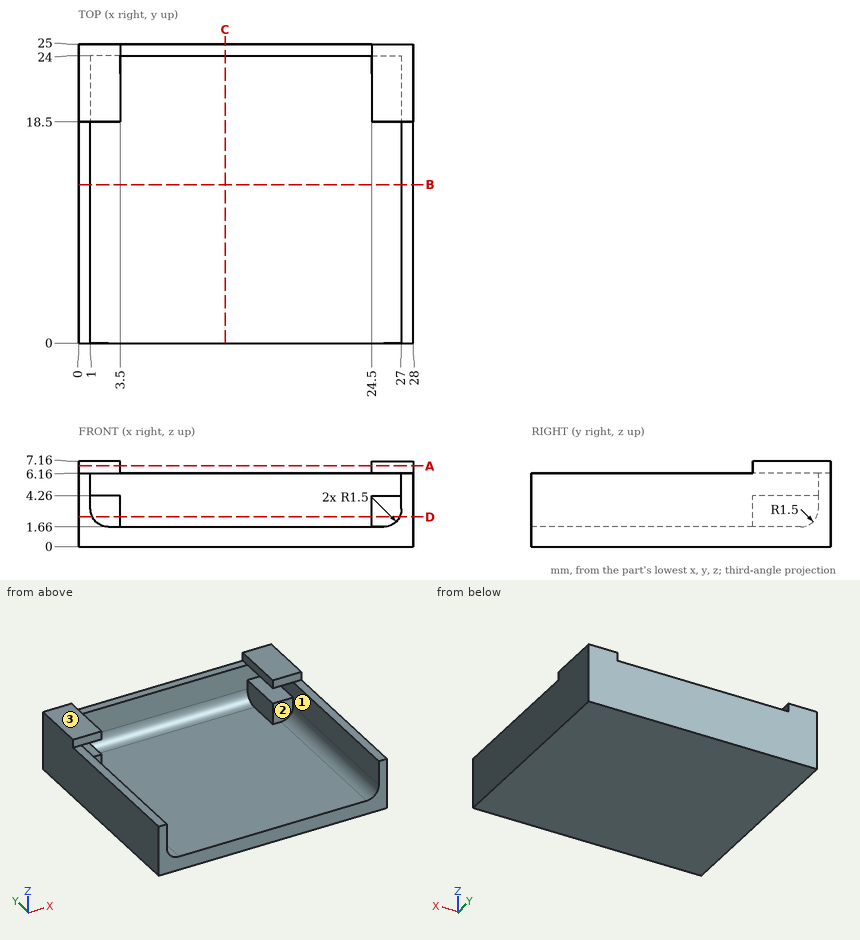
Input: dimensioned drawing with shaded views. Units: mm. Origin: part minimum x, y, z. A direction names the side the tool comes from. Coordinates: 2 decimals unless noted, no trailing zeros. Write each loop counter-clockwise with the first axis right and the second up, starting at its lowest first coordinate (ties: lowest second). Pieces come first, ordered by that corner, then holes. Notation, with made-up numbers: M -24,82 L 33,82 A23 cw 33,114 Z; hole C 80.5,24 d5. An arc over 180 degrees is marked long. Use a Markdown table: item, result.
1) Section C-C, the plane x = 12.25. Output: boundary loops of the cut face in (y, z), then the cut area to 3 significant figures.
Conclusion:
| item | result |
|---|---|
| outline | M 0,0 L 25,0 L 25,6.16 L 24,6.16 L 24,3.16 A1.5 cw 22.5,1.66 L 0,1.66 Z |
| area | 46.5 mm^2 |
2) Reachability of the marked faces 1, 2 and 3 from +Z, -Z, +X, -X, +Y, -Y: full face, straight path, thin tool, end or side. Return the list, or none.
Conclusion:
| item | result |
|---|---|
| face 1 | -Y |
| face 2 | +Z, -Y |
| face 3 | +Z, +X, -X, +Y, -Y |
3) Ray query, L1, parallel to X at y = 20.25, z = 4; L2, parallel to Y at x = 10.25, z = 3.5; L3, parallel to Y at x = 26.25, z = 3. Return the intervals inside material, ascending.
Conclusion:
| item | result |
|---|---|
| L1 | x = 0 to 3.5, 24.5 to 28 |
| L2 | y = 24 to 25 |
| L3 | y = 18.5 to 25 |
4) Section B-B, the plane y = 13.25. Output: boundary loops of the cut face in (x, z).
Conclusion:
| item | result |
|---|---|
| outline | M 0,0 L 28,0 L 28,6.16 L 27,6.16 L 27,3.16 A1.5 cw 25.5,1.66 L 2.5,1.66 A1.5 cw 1,3.16 L 1,6.16 L 0,6.16 Z |
5) Section A-A, the plane z = 6.75. Output: boundary loops of the cut face in (x, y).
Conclusion:
| item | result |
|---|---|
| outline | M 0,18.5 L 3.5,18.5 L 3.5,25 L 0,25 Z; M 24.5,18.5 L 28,18.5 L 28,25 L 24.5,25 Z |
6) First-contact query: pin 1 Ø3 at (x, z) = (6, 5) entering from -Y; pin 2 Ø0.9 at (y, z) = (15.5, 5.5) entering from -X; pin 3 Ø5 at (x, y) = (20.5, 4) entering from +Z; pin 4 Ø1.1 at (x, z) = (26.5, 6.5) entering from -Y. Flat tips, straight axial feed; report the tip coordinate or a pass-through.
Conclusion:
| item | result |
|---|---|
| pin 1 | stops at y = 24 |
| pin 2 | stops at x = 0 |
| pin 3 | stops at z = 1.66 |
| pin 4 | stops at y = 18.5 |
7) Section D-D, the plane z = 2.5. Output: boundary loops of the cut face in (x, y).
Conclusion:
| item | result |
|---|---|
| outline | M 0,0 L 1.15,0 L 1.15,18.5 L 3.5,18.5 L 3.5,23.85 L 24.5,23.85 L 24.5,18.5 L 26.85,18.5 L 26.85,0 L 28,0 L 28,25 L 0,25 Z |
